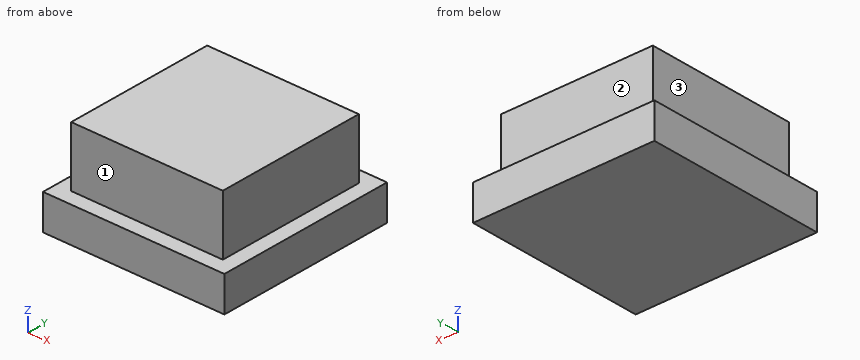
Autodesk Inventor part; units mm, degrees
ref_plane "YZ Plane" through (0, 0, 0) normal (1, 0, 0) x (0, 1, 0)
ref_plane "XZ Plane" through (0, 0, 0) normal (0, 1, 0) x (-1, 0, 0)
ref_plane "XY Plane" through (0, 0, 0) normal (0, 0, 1) x (1, 0, 0)
sketch "スケッチ1" plane through (0, 0, 0) normal (0, 0, 1) x (1, 0, 0)
  line L0 (-6.095, 6.095) -> (6.095, 6.095)
  line L1 (6.095, 6.095) -> (6.095, -6.095)
  line L2 (6.095, -6.095) -> (-6.095, -6.095)
  line L3 (-6.095, -6.095) -> (-6.095, 6.095)
  line L4 (-6.095, 6.095) -> (6.095, -6.095) construction
  line L5 (6.095, 6.095) -> (-6.095, -6.095) construction
  point P0 (0, 0)
  dimension "d0" = 12.19
  dimension "d1" = 12.19
extrude "押し出し1" add sketch "スケッチ1" along normal blind 6.35
sketch "スケッチ2" plane through (0, 0, 6.35) normal (0, 0, 1) x (1, 0, 0)
  line L0 (6.095, 6.095) -> (-6.095, 6.095)
  line L1 (-6.095, -6.095) -> (6.095, -6.095)
  line L2 (6.095, -6.095) -> (6.095, 6.095)
  line L3 (6.095, 6.095) -> (-6.095, 6.095)
  line L4 (-6.095, 6.095) -> (-6.095, -6.095)
  line L5 (-6.095, -6.095) -> (6.095, 6.095) construction
  line L6 (6.095, -6.095) -> (-6.095, 6.095) construction
  line L7 (-5.095, -5.095) -> (5.095, -5.095)
  line L8 (5.095, -5.095) -> (5.095, 5.095)
  line L9 (5.095, 5.095) -> (-5.095, 5.095)
  line L10 (-5.095, 5.095) -> (-5.095, -5.095)
  point P0 (0, 0)
  dimension "d4" = 1
extrude "押し出し2" cut sketch "スケッチ2" against normal blind 4
properties part number "Circuit_DCDCconverter_OKL-T3-W12N-C"
For this review, take the finished solid that the model builds, in its own axes (mm). Face numbers are marked on the shaded views. A direction names the side the tool comes from. Give positions to 0.01 mm unless a question says otherwise; leave off trailing zeros. Loops run counter-clockwise (first coordinate to the right, second up) from the corner with the lowest first, then second, coordinate; pieces in that order, holes last. Notation, with made-up numbers: M -15,24.5 L 16,24.5 A22 ccw 16,43.5 Z; hole C 65,-2.75 d6. An arc over 180 degrees is marked long. Put each result on its own line as item: value. Start each with the question number.
(1) Add section C-C, the plane z = 4.5. Write out the cut boundary in (x, y) (3 decimals), then the cut area to 3 significant figures.
(2) Machinability: for the marked faces 1, 2 and 3, which of the approach directions +Z, -Z, +X, -X, +Y, -Y give a long, thin tool a straight path to every point of the face, cutting with its end or side? Answer none if there is none.
(3) Wall thickness on L1, parallel to Z at x = -4.5, y = 5.75; L2, parallel to Y at x = 5, z = 3 (3 decimals): over which ranges is each line inside the solid? List them lowest first.
(4) For pin 1 (1.2 mm diameter, centred on x = 1, z = 3.5, fed in from -Y) (3 decimals); pin 2 (3 mm diameter, centred on x = 0, z = 5, fed in from +Y) (3 decimals); pin 3 (2 mm diameter, centred on y = -1, z = 4.5, fed in from -X) (3 decimals), all flat-tipped, find the tip position at first contact; note any pin that passes through.
(5) Add section A-A, the plane y = 1.25. Write out the cut boundary in (x, z) (3 decimals).
Result:
1. outline: M -5.095,-5.095 L 5.095,-5.095 L 5.095,5.095 L -5.095,5.095 Z
1. area: 104 mm^2
2. face 1: +Z, +X, -X, -Y
2. face 2: +Z, +X, -X, +Y
2. face 3: +Z, -X, +Y, -Y
3. L1: z = 0 to 2.35
3. L2: y = -5.095 to 5.095
4. pin 1: stops at y = -5.095
4. pin 2: stops at y = 5.095
4. pin 3: stops at x = -5.095
5. outline: M -6.095,0 L 6.095,0 L 6.095,2.35 L 5.095,2.35 L 5.095,6.35 L -5.095,6.35 L -5.095,2.35 L -6.095,2.35 Z
